Part print with two shaded views. Sizes in mm from the minimum x, y, z corner. Give positions to 0.01 mm unless a question says otherwise; leave off trailing zeros. Order: outer loops, then holes, each group sorted by start corner. A loop starts at its lowest first (then second) coordinate and runs counter-clockwise, first axis right, second up. Notation, with made-up numbers: (-14, 81) -> (37, 81) arc R14 cw to (37, 102) -> close; hole circle Ø6 at (30, 49). An arc over 180 degrees is marked (long way). Answer in a Markdown table with one row per item. Add a question column.
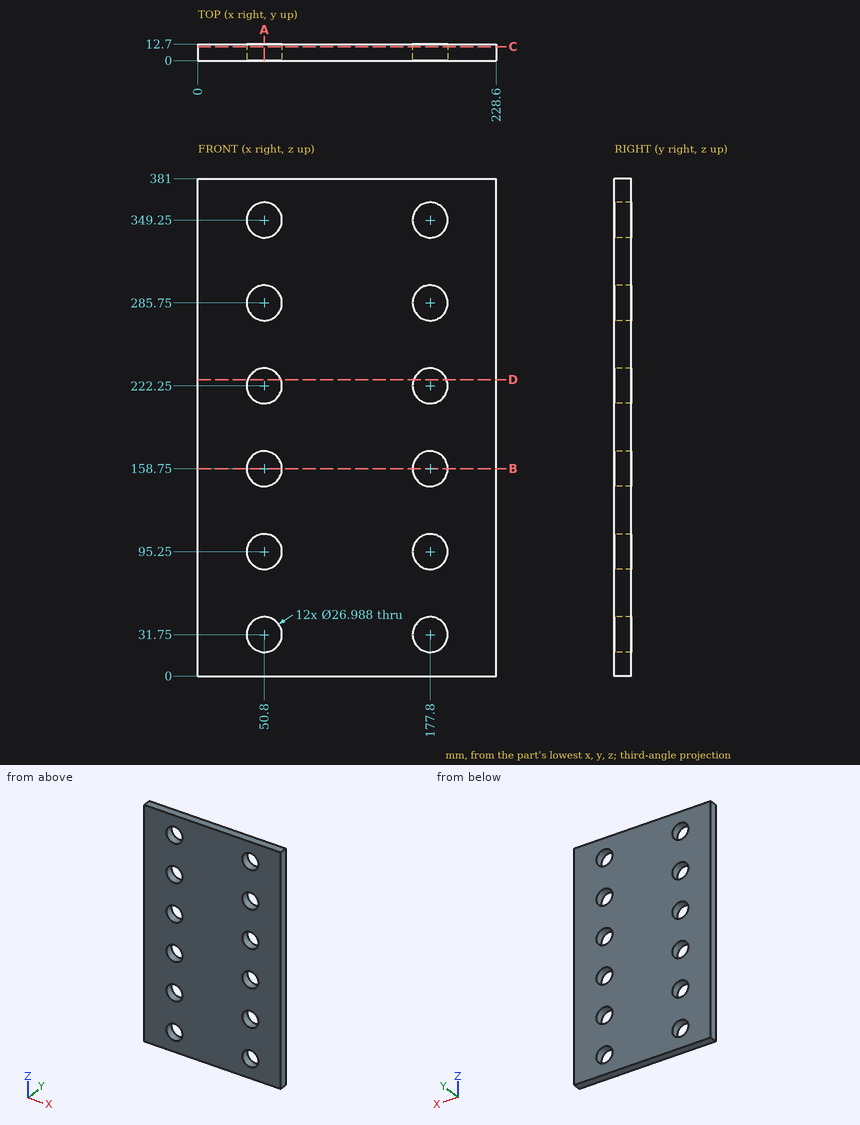
Item 1: Saw through at B-B on z = 158.75. List the corners of the cut face in (x, y).
Item 2: Wall check: line 1 (X direction, y = 4.25, z = 222.5); line 2 (X direction, y = 6.5, z = 291.5). Give the ranges that are in metal, low to high.
Item 3: Saw through at D-D on z = 227. List the corners of the cut face in (x, y), plus the area to 3 significant figures.
Item 4: Saw through at C-C on y = 10.75. Give the number of separate pieces and of enclosed holes in the cut face, plus the area to 3 significant figures.
Item 5: Saw through at A-A on x = 50.8. List the corners of the cut face in (y, z).
Evaluation:
| question | item | result |
|---|---|---|
| 1 | outline | (0, 0) -> (37.31, 0) -> (37.31, 12.7) -> (0, 12.7) -> close; (64.29, 0) -> (164.31, 0) -> (164.31, 12.7) -> (64.29, 12.7) -> close; (191.29, 0) -> (228.6, 0) -> (228.6, 12.7) -> (191.29, 12.7) -> close |
| 2 | line 1 | x = 0 to 37.31, 64.29 to 164.31, 191.29 to 228.6 |
| 2 | line 2 | x = 0 to 38.59, 63.01 to 165.59, 190.01 to 228.6 |
| 3 | outline | (0, 0) -> (38.17, 0) -> (38.17, 12.7) -> (0, 12.7) -> close; (63.43, 0) -> (165.17, 0) -> (165.17, 12.7) -> (63.43, 12.7) -> close; (190.43, 0) -> (228.6, 0) -> (228.6, 12.7) -> (190.43, 12.7) -> close |
| 3 | area | 2,260 mm2 |
| 4 | separate pieces | 1 |
| 4 | enclosed holes | 12 |
| 4 | area | 80,200 mm2 |
| 5 | outline | (0, 0) -> (12.7, 0) -> (12.7, 18.26) -> (0, 18.26) -> close; (0, 45.24) -> (12.7, 45.24) -> (12.7, 81.76) -> (0, 81.76) -> close; (0, 108.74) -> (12.7, 108.74) -> (12.7, 145.26) -> (0, 145.26) -> close; (0, 172.24) -> (12.7, 172.24) -> (12.7, 208.76) -> (0, 208.76) -> close; (0, 235.74) -> (12.7, 235.74) -> (12.7, 272.26) -> (0, 272.26) -> close; (0, 299.24) -> (12.7, 299.24) -> (12.7, 335.76) -> (0, 335.76) -> close; (0, 362.74) -> (12.7, 362.74) -> (12.7, 381) -> (0, 381) -> close |
